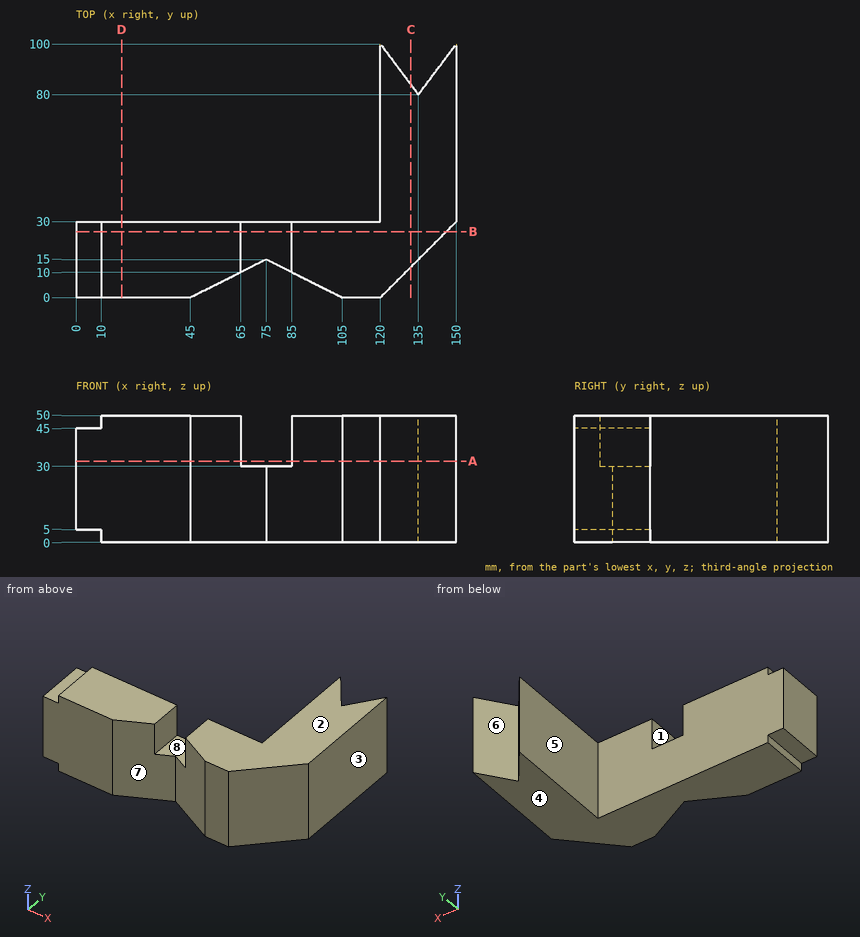
Source: three-view drawing plus pictorial views. Frame: mm from the lowest corner of the part. A direction names the side the tool comes from. Coordinates: 2 decimals unless noted, no trailing zeros. Loops run counter-clockwise (first coordinate to the right, second up) from the corner with the lowest first, then second, coordinate; pieces in that order, holes last. Notation, with made-up numbers: (-2, 56) -> (54, 56) arc R22 ccw to (54, 63) -> close; hole circle Ø7 at (-21.75, 4.25). An arc over 180 degrees is marked (long way). Write each question's results on one line, items separated by ' | '. Start each with the question number.
Q1. Section C-C, the plane x = 132. Return the cut outline in (y, z).
Q2. Ray query, line 1 (X direction, y = 28, z = 39.5); line 2 (X direction, y = 60, z = 44.5); line 3 (X direction, y = 88, z = 24). Return the intervals inside material, ascending. Write a range as from..to.
Q3. Section B-B, the plane y = 26. Return the cut outline in (x, z).
Q4. Section A-A, the plane z = 32. Return the cut outline in (x, y), plus the area to 3 significant figures.
Q5. Pull-direction query (X, two-part tool) for the marked faces 1, 2 and 3; classes: released by +X, released by -X, zero draft, split by the parting line, or undercut.
Q6. Pin query (flat end, axial travel): pin 1 (4 mm diameter, centred on y = 13, z = 48, fed in from -X); pin 2 (10 mm diameter, centred on x = 77.5, y = 20, fed in from +Z); pin 3 (8 mm diameter, centred on x = 3, y = 19, fed in from -Z). Return the tip coordinate at first contact, or that it passes through.
Q7. Section D-D, the plane x = 18. Return the cut outline in (y, z), plus the area to 3 significant figures.
Q8. Reachability of the marked faces 4, 5, 6, 7 and 8 from +Z, -Z, +X, -X, +Y, -Y: full face, straight path, thin tool, end or side. Return the list, or none.
Found:
1) outline: (12, 0) -> (84, 0) -> (84, 50) -> (12, 50) -> close
2) line 1: 0..65, 85..148 | line 2: 120..150 | line 3: 120..129, 141..150
3) outline: (0, 5) -> (10, 5) -> (10, 0) -> (146, 0) -> (146, 50) -> (85, 50) -> (85, 30) -> (65, 30) -> (65, 50) -> (10, 50) -> (10, 45) -> (0, 45) -> close
4) outline: (0, 0) -> (45, 0) -> (65, 10) -> (65, 30) -> (0, 30) -> close; (85, 10) -> (105, 0) -> (120, 0) -> (150, 30) -> (150, 100) -> (135, 80) -> (120, 100) -> (120, 30) -> (85, 30) -> close | area: 5,050 mm2
5) face 1: undercut | face 2: zero draft | face 3: released by +X
6) pin 1: x = 10 | pin 2: z = 30 | pin 3: z = 5
7) outline: (0, 0) -> (30, 0) -> (30, 50) -> (0, 50) -> close | area: 1,500 mm2
8) face 4: -Z, +X, -X, +Y, -Y | face 5: +Z, -Z, -X, +Y | face 6: +Z, -Z, +Y | face 7: +Z, -Z, -Y | face 8: +Z, +Y, -Y
